```python
from build123d import *

# Parameters (mm, degrees)
BOSS_EXTRUDE1_DEPTH      = 50.8
BOSS_EXTRUDE1_DEPTH_BACK = 3.556
SKETCH2_R                = 12.7
SKETCH2_R_2              = 7.9375


with BuildPart() as part:
    # Sketch1 → Revolve1 (revolve)
    with BuildSketch(Plane.XY, mode=Mode.PRIVATE) as revolve1_sk:
        with BuildLine():
            Line((-166.116, -123.571), (-55.372, -123.571))
            add(Edge.make_bspline(
                [(-55.372, -123.571), (0, -123.571), (0, 0)],
                knots=[3.141592654, 3.141592654, 3.141592654, 4.71238898, 4.71238898, 4.71238898], degree=2, weights=[1, 0.707106781, 1]))
            Line((0, 0), (-14.224, 0))
            add(Edge.make_bspline(
                [(-55.372, -109.347), (-14.224, -109.347), (-14.224, 0)],
                knots=[0, 0, 0, 1.570796327, 1.570796327, 1.570796327], degree=2, weights=[1, 0.707106781, 1]))
            Line((-55.372, -109.347), (-166.116, -109.9185))
            Line((-166.116, -109.9185), (-166.116, -123.571))
        make_face()
    revolve(revolve1_sk.sketch.rotate(Axis((-166.116, 0, 0), (1, 0, 0)), 270), axis=Axis((-166.116, 0, 0), (1, 0, 0)))

    # Sketch2 → Boss-Extrude1 (add, two sides: drawn at the far end of the back side and taken through both)
    with BuildSketch(Plane(origin=(0, 0, 0), x_dir=(0, 0, -1), z_dir=(1, 0, 0)).offset(-BOSS_EXTRUDE1_DEPTH_BACK)):
        Circle(SKETCH2_R)
        Circle(SKETCH2_R_2, mode=Mode.SUBTRACT)
    extrude(amount=BOSS_EXTRUDE1_DEPTH + BOSS_EXTRUDE1_DEPTH_BACK)


solid = part.part
```
The listing builds one solid part. Answer for the finished solid, in the listing's coordinates (mm). A direction names the side the tool comes from. Give positions to 0.01 mm unless a question says otherwise; leave off trailing zeros. Write each loop counter-clockwise with the first axis right and the second up, starting at its lowest first coordinate (ties: lowest second). Pieces come first, ordered by that corner, then holes. Notation, with made-up numbers: M 42,-12.75 L 77,-12.75 A21 ccw 77,25.25 Z; hole C 48,-31.5 d3. An arc over 180 degrees is marked long. Write each question's results on one line, items separated by ' | '.
Q1. For a pull along Z with two mould halves and no side action, classify faces 1 (the flat face through (50.8, -8.3, 0.2)), 2 (the conical face through (-111.52, 107.03, -23.77)), 3 (the cylindrical face through (-109.969, -83.515, -91.077)) as released by +Z, released by -Z, zero draft, split by the parting line, or undercut.
Output values:
face 1: zero draft | face 2: undercut | face 3: split by the parting line
Q2. Flat-ended cylindrical pins translate along their axes: P1, Ø6, axis at x = -108.5, y = 37.5, coming from the -Z side; P2, Ø8, axis at y = 18, z = 32.5, coming from the -X side; P3, Ø8, axis at y = -29, z = -4.5, coming from the -X side. Find the tip coordinate at first contact, or state that the pin passes through.
Output values:
P1: z = -118.66 | P2: x = -17.25 | P3: x = -16.18
Q3. A tool of negligible diameter and unlimited length cuts with its end or side. For faces 4 (the cylindrical face through (24.9, -12.4, 2.75)), 5 (the flat face through (-166.116, 73, 83)), from which of +Z, -Z, +X, -X, +Y, -Y can it reach the whole face along a straight path? Write none if from no direction.
Output values:
face 4: +X | face 5: +Z, -Z, -X, +Y, -Y
Q4. Section A-A, the plane x = 12 is taken. Write down the section's boundary in (y, z) (1 decimal), then the cut area to 3 significant figures.
Output values:
outline: C 0,0 d25.4; hole C 0,0 d15.9 | area: 309 mm2
Q5. Section B-B, the plane x = -138 is taken. Write down the section's boundary in (y, z), then the cut area to 3 significant figures.
Output values:
outline: C 0,0 d247.14; hole C 0,0 d219.55 | area: 10,100 mm2
Q6. Consider L1, parallel to Y at x = 18, z = 0; L2, parallel to Y at x = -118, z = 70.5; L3, parallel to Z at x = -56, y = 34.5. Determine where each line is inside the solid, lowest interval first. Write a range as from..to.
Output values:
L1: -12.7..-7.94, 7.94..12.7 | L2: -101.49..-84.01, 84.01..101.49 | L3: -118.66..-103.77, 103.77..118.66
